Could you check a few things on this drawing? It's one solid part, dimensions in mm from its lowest x, y, z. A direction names the side the tool comes from. Coordinates: 2 decimals unless noted, no trailing zeros. Write each loop counter-clockwise with the first axis right and the second up, starting at its lowest first coordinate (ties: lowest second). Pieces come first, ordered by that corner, then holes. Notation, with made-up numbers: (56, 70) - (63, 70) arc R18 ccw to (63, 78) - close; hole circle Ø9 at (-24, 27.25). An arc over 180 degrees is marked (long way). Answer as a JSON object with one key per item and string values. Group by question number.
1) We'd pull the mould along Y, two halves only. Please class the marked faces 1, 2, 3 and 4: released by +Y, released by -Y, zero draft, split by the parting line, or undercut.
2) Will this pin go through, and if not, where does the flat tip stop? pin 1 Ø3 at (x, y) = (7.62, 30.92) entering from -Z.
3) If we section it at A-A (x = 3.81): Write out the boundary of the cut face in (y, z) (1 decimal).
4) If we section it at C-C (x = 11): Write out the boundary of the cut face in (y, z) (1 decimal).
5) If we section it at B-B (z = 14.25): Write out the boundary of the cut face in (x, y) (1 decimal), plus the area to 3 significant figures.
6) On a 3-axis mill with a long thin cutter (end or side, diameter ignored), from which of +Z, -Z, +X, -X, +Y, -Y can I reach the whole of each face in a straight line? I mean the marked faces 5 and 6. Say none if no direction works.
7) Please list where these lines run through material, in increasing order: line 1 along Y through (x, z) = (11.25, 21.25) (1 decimal); line 2 along Y through (x, z) = (4, 14.5) (1 decimal); line 3 along Y through (x, z) = (3.81, 18.5) (1 decimal).
8) If we section it at D-D (z = 6): Write out the boundary of the cut face in (x, y).
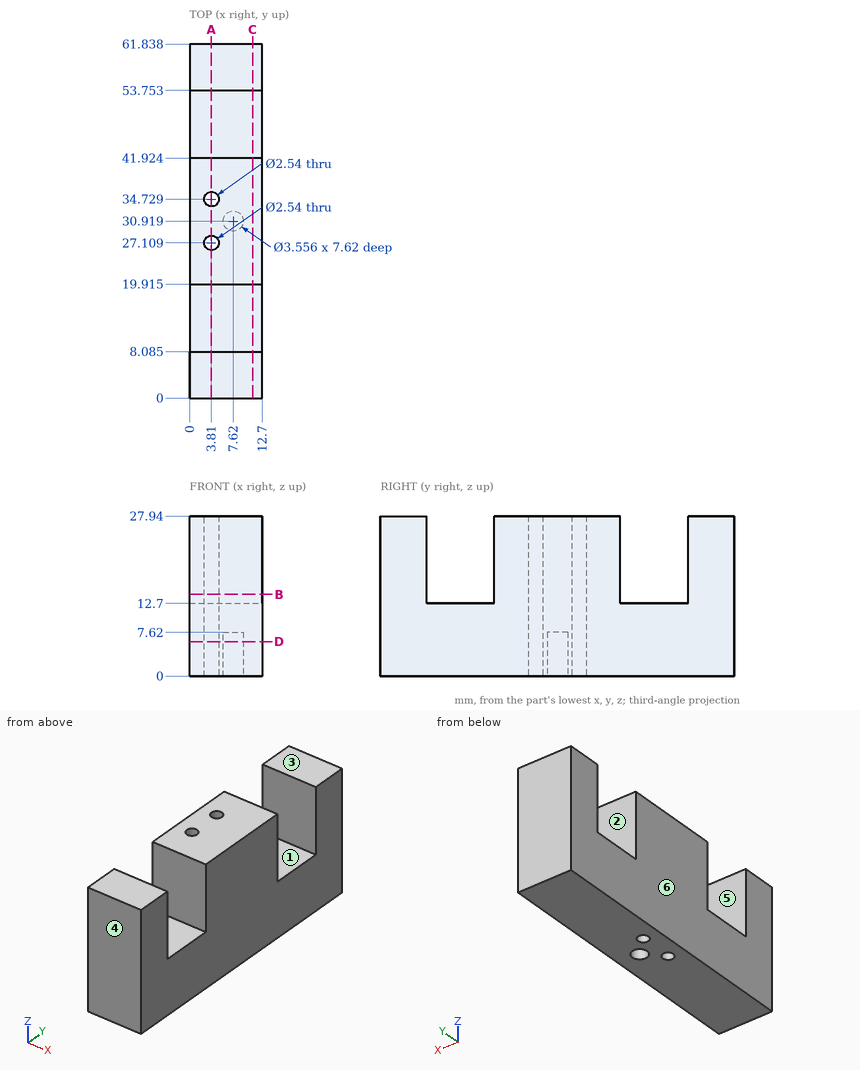
Here are the results:
{
 "1": {"face 1": "undercut", "face 2": "undercut", "face 3": "zero draft", "face 4": "released by -Y"},
 "2": {"pin 1": "stops at z = 7.62"},
 "3": {"outline": "(0, 0) - (25.8, 0) - (25.8, 27.9) - (19.9, 27.9) - (19.9, 12.7) - (8.1, 12.7) - (8.1, 27.9) - (0, 27.9) - close; (28.4, 0) - (33.5, 0) - (33.5, 27.9) - (28.4, 27.9) - close; (36, 0) - (61.8, 0) - (61.8, 27.9) - (53.8, 27.9) - (53.8, 12.7) - (41.9, 12.7) - (41.9, 27.9) - (36, 27.9) - close"},
 "4": {"outline": "(0, 0) - (61.8, 0) - (61.8, 27.9) - (53.8, 27.9) - (53.8, 12.7) - (41.9, 12.7) - (41.9, 27.9) - (19.9, 27.9) - (19.9, 12.7) - (8.1, 12.7) - (8.1, 27.9) - (0, 27.9) - close"},
 "5": {"outline": "(0, 0) - (12.7, 0) - (12.7, 8.1) - (0, 8.1) - close; (0, 19.9) - (12.7, 19.9) - (12.7, 41.9) - (0, 41.9) - close; (0, 53.8) - (12.7, 53.8) - (12.7, 61.8) - (0, 61.8) - close; hole circle Ø2.5 at (3.8, 27.1); hole circle Ø2.5 at (3.8, 34.7)", "area": "475 mm²"},
 "6": {"face 5": "+Z, +X, -X", "face 6": "+Z, -Z, -X, +Y, -Y"},
 "7": {"line 1": "y = 0 to 8.1, 19.9 to 41.9, 53.8 to 61.8", "line 2": "y = 0 to 8.1, 19.9 to 25.9, 28.4 to 33.5, 36 to 41.9, 53.8 to 61.8", "line 3": "y = 0 to 8.1, 19.9 to 25.8, 28.4 to 33.5, 36 to 41.9, 53.8 to 61.8"},
 "8": {"outline": "(0, 0) - (12.7, 0) - (12.7, 61.84) - (0, 61.84) - close; hole circle Ø2.54 at (3.81, 27.11); hole circle Ø2.54 at (3.81, 34.73); hole circle Ø3.56 at (7.62, 30.92)"}
}
